from build123d import *

# Parameters (mm, degrees)
SKETCH1_R           = 16.5
SKETCH1_R_2         = 13.5
SKETCH4_R           = 16.5
SKETCH4_R_2         = 13.5
BOSS_EXTRUDE2_DEPTH = 40


with BuildPart() as part:
    # Sweep2: sweep along a path in Sketch3
    with BuildLine(Plane.XY) as sweep2_path:
        Line((0, 0), (0, 80))
    # Sketch1 → Sweep2 (sweep)
    with BuildSketch(Plane(origin=(0, 0, 0), x_dir=(1, 0, 0), z_dir=(0, 1, 0))):
        Circle(SKETCH1_R)
        Circle(SKETCH1_R_2, mode=Mode.SUBTRACT)
    sweep(path=sweep2_path.line)

    # Sketch4 → Boss-Extrude2 (add)
    with BuildSketch(Plane.XY):
        with Locations((0, 40)):
            Circle(SKETCH4_R)
        with Locations((0, 40)):
            Circle(SKETCH4_R_2, mode=Mode.SUBTRACT)
    extrude(amount=BOSS_EXTRUDE2_DEPTH)


solid = part.part
Could you check a few things on this model? Use its own coordinates, in mm. A direction names the side the tool comes from. Give positions to 0.01 mm unless a question says otherwise; leave off trailing zeros. Order: outer loops, then holes, each group sorted by start corner. A loop starts at its lowest first (then second) coordinate and runs counter-clockwise, first axis right, second up. Notation, with made-up numbers: (35, 89.25) -> (89, 89.25) arc R9 ccw to (89, 95.25) -> close; hole circle Ø8 at (32, 70.25). An arc over 180 degrees is marked (long way). Answer in a Markdown table with one row per item. Add a question column.
Item 1: Imagine slicing it at C-C (y = 21.5). List the corners of the cut face in (x, z) for me, and give its area (3 significant figures).
Item 2: For faces 1 (the cylindrical face through (12.47, 34.83, 27.92)), 2 (the flat face through (1, 54, 0)), 3 (the cylindrical face through (0.297, 53.497, 5.156)), which set-ups out of +Z, -Z, +X, -X, +Y, -Y let a thin tool reach every point of the face, with its end or its side?
Item 3: Please list where these lines run through material, in increasing order: probe 1 along X at (y, z) = (40, 33.5); probe 2 along X at (y, z) = (54, 6.5); probe 3 along Y at (x, z) = (0, 18).
Item 4: Imagine slicing it at A-A (x = 0). List the corners of the cut face in (y, z) for me, and give its area (3 significant figures).
Item 5: I'm going to push flat-ended pins straight in: P1, Ø4, axis at y = 23.5, z = 31, coming from the +X side; P2, Ø1.5, axis at x = -7, z = -1, coming from the -Y side; P3, Ø5, axis at x = -5.5, z = 28, coming from the -Y side (3 decimals); P4, Ø8, axis at y = 71.5, z = -8.5, coming from the -X side. Where does each tip first touch, or does it pass through?
Item 6: We'd pull the mould along Y, two halves only. Please class faces 4 (the cylindrical face through (-0.297, 26.503, 5.156)), 5 (the cylindrical face through (7.61, 25.36, 24.16)), 6 (the flat face through (0, 0, -14)): pulls with the +Y half, pulls with the -Y half, needs draft (parallel to the pull), parting line crosses it, or undercut.
Item 7: Imagine slicing it at D-D (z = -4). List the corners of the cut face in (x, y) for me.
Item 8: Imagine slicing it at B-B (z = 7). List the corners of the cut face in (x, y) for me, and give its area (3 significant figures).
Result:
| question | item | result |
|---|---|---|
| 1 | outline | circle Ø33 at (0, 0); hole circle Ø27 at (0, 0) |
| 1 | area | 283 mm2 |
| 2 | face 1 | +Z |
| 2 | face 2 | +Y, -Y |
| 2 | face 3 | none |
| 3 | probe 1 | -16.5 to -13.5, 13.5 to 16.5 |
| 3 | probe 2 | -15.17 to -11.83, -8.73 to 8.73, 11.83 to 15.17 |
| 3 | probe 3 | 23.5 to 26.5, 53.5 to 56.5 |
| 4 | outline | (0, -16.5) -> (80, -16.5) -> (80, -13.5) -> (0, -13.5) -> close; (0, 13.5) -> (23.5, 13.5) -> (23.5, 0) -> (26.5, 0) -> (26.5, 13.5) -> (53.5, 13.5) -> (53.5, 0) -> (56.5, 0) -> (56.5, 13.5) -> (80, 13.5) -> (80, 16.5) -> (56.5, 16.5) -> (56.5, 40) -> (53.5, 40) -> (53.5, 16.5) -> (26.5, 16.5) -> (26.5, 40) -> (23.5, 40) -> (23.5, 16.5) -> (0, 16.5) -> close |
| 4 | area | 702 mm2 |
| 5 | P1 | x = 7.87 |
| 5 | P2 | through |
| 5 | P3 | y = 23.775 |
| 5 | P4 | x = -15.87 |
| 6 | face 4 | undercut |
| 6 | face 5 | parting line crosses it |
| 6 | face 6 | pulls with the -Y half |
| 7 | outline | (-16.01, 0) -> (-12.89, 0) -> (-12.89, 80) -> (-16.01, 80) -> close; (12.89, 0) -> (16.01, 0) -> (16.01, 80) -> (12.89, 80) -> close |
| 8 | outline | (-14.94, 0) -> (-11.54, 0) -> (-11.54, 28.21) arc R16.5 ccw to (11.54, 28.21) -> (11.54, 0) -> (14.94, 0) -> (14.94, 33) arc R16.5 ccw to (14.94, 47) -> (14.94, 80) -> (11.54, 80) -> (11.54, 51.79) arc R16.5 ccw to (-11.54, 51.79) -> (-11.54, 80) -> (-14.94, 80) -> (-14.94, 47) arc R16.5 ccw to (-14.94, 33) -> close; hole (-11.54, 33) arc R13.5 ccw to (11.54, 33) -> (11.54, 47) arc R13.5 ccw to (-11.54, 47) -> close |
| 8 | area | 732 mm2 |
